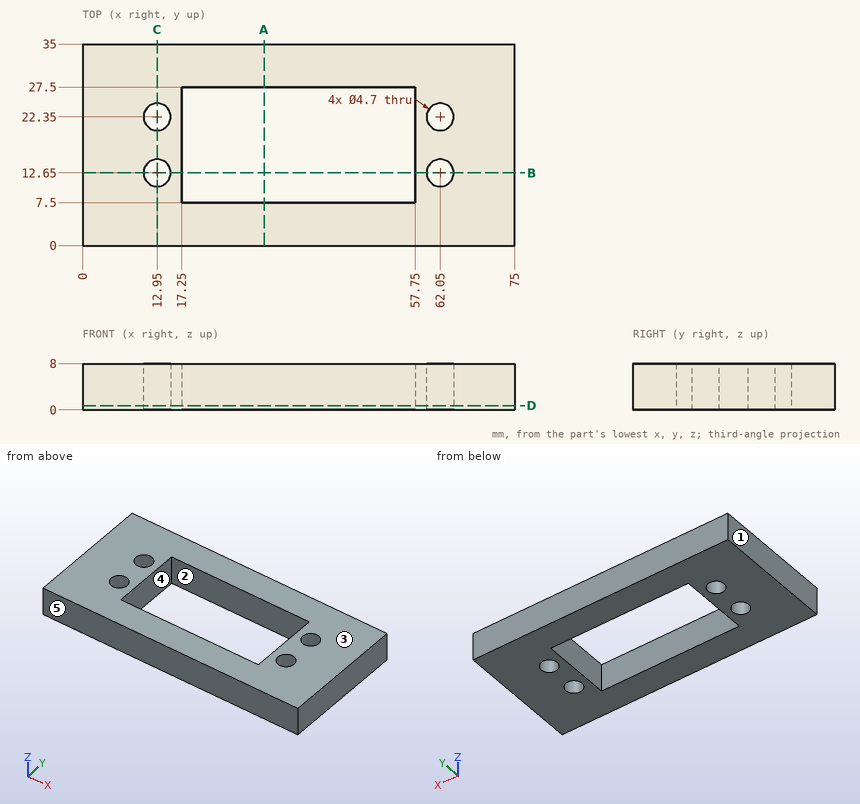
Print and shaded views of the part. All mm, measured from the part's lowest x, y and z. A direction names the side the tool comes from. Round coordinates to 2 decimals unless told otherwise and drop trailing zeros. Write each loop counter-clockwise with the first axis right and the second up, starting at its lowest first coordinate (ties: lowest second). Pieces come first, ordered by that corner, then holes. Notation, with made-up numbers: (73, 81.5) -> (121, 81.5) arc R15 ccw to (121, 88.5) -> close; hole circle Ø11 at (4, 1.25). An arc over 180 degrees is marked (long way). Write item = value, one per line.
(1) Tool access for the marked faces 4 and 5: list every direction of +Z, -Z, +X, -X, +Y, -Y with a clear straight run to the whole face (end or side of a thin tool).
Answer:
face_4 = +Z, -Z
face_5 = +Z, -Z, +X, -X, -Y
(2) Probe L1, parallel to Y at x = 12.95, z = 2.75; L2, parallel to X at y = 22.5, z = 5.75; L3, parallel to X at y = 16.5, z = 4. List the from-to ranges inside material, lowest first.
Answer:
L1 = 0 to 10.3, 15 to 20, 24.7 to 35
L2 = 0 to 10.6, 15.3 to 17.25, 57.75 to 59.7, 64.4 to 75
L3 = 0 to 17.25, 57.75 to 75
(3) Band-saw the part on A-A (x = 31.5). Give the cut face in (y, z).
Answer:
outline = (0, 0) -> (7.5, 0) -> (7.5, 8) -> (0, 8) -> close; (27.5, 0) -> (35, 0) -> (35, 8) -> (27.5, 8) -> close
(4) Two-plate mould, pull along X, no slides. Class the marked faces 1, 2 and 3: pulls with the +X half, pulls with the -X half, needs draft (parallel to the pull), parting line crosses it, or undercut.
Answer:
face_1 = pulls with the -X half
face_2 = undercut
face_3 = needs draft
(5) Flat gauge pin, fed straight in: pin 1 (1 mm diameter, centred on x = 14, y = 20.5, fed in from -Z). Where does the tip first touch, or does it go through?
Answer:
pin_1 = 0
(6) Band-saw the part on C-C (x = 12.95). Give the cut face in (y, z).
Answer:
outline = (0, 0) -> (10.3, 0) -> (10.3, 8) -> (0, 8) -> close; (15, 0) -> (20, 0) -> (20, 8) -> (15, 8) -> close; (24.7, 0) -> (35, 0) -> (35, 8) -> (24.7, 8) -> close
(7) Band-saw the part on B-B (y = 12.65). Give the cut face in (x, z), then the cut area to 3 significant figures.
Answer:
outline = (0, 0) -> (10.6, 0) -> (10.6, 8) -> (0, 8) -> close; (15.3, 0) -> (17.25, 0) -> (17.25, 8) -> (15.3, 8) -> close; (57.75, 0) -> (59.7, 0) -> (59.7, 8) -> (57.75, 8) -> close; (64.4, 0) -> (75, 0) -> (75, 8) -> (64.4, 8) -> close
area = 201 mm2
(8) Band-saw the part on D-D (z = 0.75). Give the cut face in (x, y), then the cut area to 3 significant figures.
Answer:
outline = (0, 0) -> (75, 0) -> (75, 35) -> (0, 35) -> close; hole circle Ø4.7 at (12.95, 12.65); hole circle Ø4.7 at (12.95, 22.35); hole (17.25, 7.5) -> (57.75, 7.5) -> (57.75, 27.5) -> (17.25, 27.5) -> close; hole circle Ø4.7 at (62.05, 12.65); hole circle Ø4.7 at (62.05, 22.35)
area = 1,750 mm2
